Drawing for the job (mm, zero at the part's lowest x, y, z). Round coordinates to 2 decimals unless told otherwise and drop trailing zeros. Order: outer loops, then holes, each group sorted by start corner. A loop starts at its lowest first (then second) coordinate and runs counter-clockwise, first axis right, second up. Notation, with made-up numbers: (23, -38.75) - (65, -38.75) arc R8 ccw to (65, -27.75) - close; hole circle Ø5 at (-26, 31). An arc over 180 degrees is marked (long way). Answer as a JSON object with one key per item and string values.
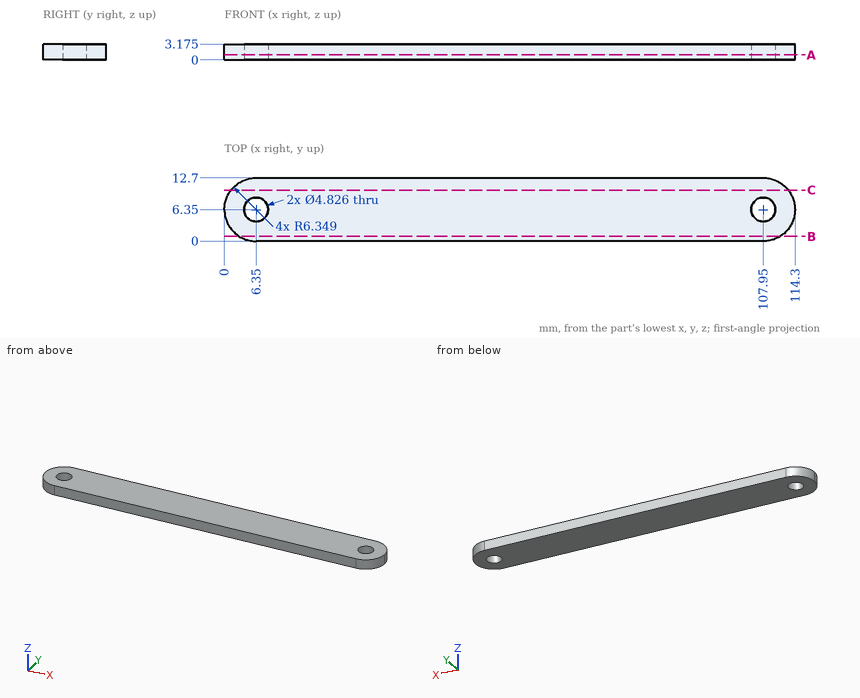
Item 1: Cut at B-B (y = 1). Write the cut outline in (x, z) (1 decimal).
Taken from the geometry:
{"outline": "(2.9, 0) - (111.4, 0) - (111.4, 3.2) - (2.9, 3.2) - close"}
Item 2: Probe L1, parallel to X at y = 6.35, z = 1.15; L2, parallel to Y at x = 107.95, z = 1.3; L3, parallel to X at y = 4.5, z = 0.3 (1 decimal). List the from-to ranges inside material, lowest first. Write a range as from..to.
Taken from the geometry:
{"L1": "0..3.94, 8.76..105.54, 110.36..114.3", "L2": "0..3.94, 8.76..12.7", "L3": "0.3..4.8, 7.9..106.4, 109.5..114"}
Item 3: Cut at C-C (y = 10.25). Write the cut outline in (x, z) (1 decimal).
Taken from the geometry:
{"outline": "(1.3, 0) - (113, 0) - (113, 3.2) - (1.3, 3.2) - close"}
Item 4: Cut at A-A (z = 1). State how many separate pieces and enclosed holes the cut face has, plus the area to 3 significant figures.
Taken from the geometry:
{"separate pieces": "1", "enclosed holes": "2", "area": "1,380 mm2"}
